Input: part model. Units: mm. Frame: model coordinates. A direction names the side the tool comes from. Round coordinates to 2 decimals unless told otherwise and drop trailing zeros. Loops run counter-clockwise (first coordinate to the right, second up) from the corner with the lowest first, then second, coordinate; pieces in that order, holes last. Notation, with made-up numbers: M 74.25,-14.5 L 82.25,-14.5 A29 cw 82.25,23.5 Z; hole C 68.5,-40 d2. An arc over 180 degrees is marked long. Use one line per item in the form item = value. Start each with the question number.
Q1. Access query for faces 5 (the flat face through (-6, 1.016, -70)), 6 (the flat face through (-6, 7, 0)). Directions: +Z, -Z, +X, -X, +Y, -Y. A direction counts if a zero-diameter tool reaches every point of the face in a straight line with its end or side. Return the directions, or none.
Q2. Section query B-B, the plane x = -6.25. Output: boundary loops of the cut face in (y, z) (3 decimals), and give its area (3 significant figures).
Q3. Mould query, pull axis Y, two halves, no side actions, for faces 1 (the cylindrical face through (-5.242, 9.311, -70.437)), 2 (the cylindrical face through (-8.952, 4.906, -70.437)), 3 (the flat face through (-6, 7, -142.875)), 4 (the cylindrical face through (-4.447, 8.666, -70.437)). Classes: pulls with the +Y half, pulls with the -Y half, needs draft (parallel to the pull), parting line crosses it, or undercut.
Q4. Section query A-A, the plane z = -128.5. Output: boundary loops of the cut face in (x, y) (1 decimal), and give its area (3 significant figures).
Q5. First-contact query: P1, Ø0.7, axis at y = 4, z = -68.5, coming from the -X side; P2, Ø1, axis at y = 12, z = -79, coming from the +X side; P3, Ø2, axis at y = 10, z = -82, coming from the +X side. Flat tips, straight axial feed; report the tip coordinate or a pass-through.
Q6. Ray query, line 1 along Y through (x, z) = (-11.25, -63.5) (3 decimals); line 2 along Y through (x, z) = (-2.75, -43.5); line 3 along X through (y, z) = (1.75, -133). Return the intervals inside material, ascending.
```python
from build123d import *

# Parameters (mm, degrees)
EXTRUDE_THIN1_DEPTH = 142.875
FILLET1_R           = 1.016


with BuildPart() as part:
    # Sketch1 → Extrude-Thin1 (new body)
    with BuildSketch(Plane.XY):
        with BuildLine():
            Line((-0.396875, 11.137402345), (0, 14.2875))
            Line((0, 14.2875), (-3.96875, 14.2875))
            ThreePointArc((-3.96875, 14.2875), (-5.03336677, 9.671261516), (-8.352026926, 6.290498085))
            ThreePointArc((-8.352026926, 6.290498085), (-9.684272791, 5.742948706), (-11.1125, 5.55625))
            Line((-11.1125, 5.55625), (-11.1125, 3.175))
            Line((-11.1125, 3.175), (-12.7, 3.175))
            Line((-12.7, 3.175), (-12.7, 0))
            Line((-12.7, 0), (-0.396875, 0))
            Line((-0.396875, 0), (-0.396875, 1.016))
            Line((-0.396875, 1.016), (-11.684, 1.016))
            Line((-11.684, 1.016), (-11.684, 2.159))
            Line((-11.684, 2.159), (-10.0965, 2.159))
            Line((-10.0965, 2.159), (-10.0965, 4.619256276))
            ThreePointArc((-10.0965, 4.619256276), (-8.935783532, 4.911179537), (-7.847254707, 5.408760591))
            ThreePointArc((-7.847254707, 5.408760591), (-4.411092734, 8.723027869), (-2.960927924, 13.2715))
            Line((-2.960927924, 13.2715), (-1.152035714, 13.2715))
            Line((-1.152035714, 13.2715), (-1.40490625, 11.264402345))
            Line((-1.40490625, 11.264402345), (-0.396875, 11.137402345))
        make_face()
    extrude(amount=-EXTRUDE_THIN1_DEPTH)

    # Fillet1
    fillet1_edges = [part.edges().sort_by_distance(p)[0] for p in [
        (-10.0965, 2.159, -71.4375),
        (-12.7, 0, -71.4375),
        (-12.7, 3.175, -71.4375),
        (-11.1125, 5.55625, -71.4375),
        (-3.96875, 14.2875, -71.4375),
    ]]
    fillet(fillet1_edges, radius=FILLET1_R)


solid = part.part
```
Results found:
q1.face_5 = +Z, -Z, +X
q1.face_6 = +Z, +X, -X, +Y, -Y
q2.outline = M 0,-142.875 L 1.016,-142.875 L 1.016,0 L 0,0 Z; M 6.551,-142.875 L 7.972,-142.875 L 7.972,0 L 6.551,0 Z
q2.area = 348 mm²
q3.face_1 = pulls with the +Y half
q3.face_2 = undercut
q3.face_3 = needs draft
q3.face_4 = undercut
q4.outline = M -12.7,1 A1 ccw -11.7,0 L -0.4,0 L -0.4,1 L -11.7,1 L -11.7,2.2 L -11.1,2.2 A1 ccw -10.1,3.2 L -10.1,4.6 A6.6 ccw -7.8,5.4 A9.7 ccw -3,13.3 L -1.2,13.3 L -1.4,11.3 L -0.4,11.1 L 0,14.3 L -3,14.3 A1 ccw -4,13.3 A8.7 cw -8.4,6.3 A5.6 cw -10.3,5.6 A1 ccw -11.1,4.6 L -11.1,3.2 L -11.7,3.2 A1 ccw -12.7,2.2 Z
q4.area = 35.2 mm²
q5.P1 = -11.11
q5.P2 = -0.23
q5.P3 = -3.37
q6.line_1 = 0 to 1.016, 2.159 to 3.175
q6.line_2 = 0 to 1.02, 13.27 to 14.29
q6.line_3 = -12.7 to -11.68
